Build history of the part. All positions in model axes, mm. Round coordinates to 2 decimals unless told otherwise and drop trailing zeros. Loops run counter-clockwise (first coordinate to the right, second up) from the corner with the lowest first, then second, coordinate; pieces in that order, holes last. Notation, with made-up numbers: (72, 20) - (110, 20) arc R28 cw to (110, 43) - close; hole circle Ø2 at (70.5, -6.5). An arc over 180 degrees is marked (long way). Use a Markdown table: item, result.
from build123d import *

# Parameters (mm, degrees)
F0_W     = 254
F0_H     = 254
F1_DEPTH = 162.56
F2_R     = 60.882574
F3_DEPTH = 289.56
F4_SIZE  = 5.08
F5_R     = 12.7
F6_R     = 12.7


with BuildPart() as f1:
    # F0 (on Top) → F1 (new body)
    with BuildSketch(Plane.XY):
        Rectangle(F0_W, F0_H)
    extrude(amount=F1_DEPTH)

    # F2 (on face) → F3 (cut)
    with BuildSketch(Plane.XY.offset(162.56)):
        Circle(F2_R)
    extrude(amount=-F3_DEPTH, mode=Mode.SUBTRACT)

    # F4
    f4_edges = [f1.edges().sort_by_distance(p)[0] for p in [
        (127, 0, 162.56),
        (0, -127, 162.56),
        (-127, 0, 162.56),
        (0, 127, 162.56),
        (-60.882574, 0, 162.56),
    ]]
    chamfer(f4_edges, length=F4_SIZE)

    # F5
    f5_edges = [f1.edges().sort_by_distance(p)[0] for p in [
        (-127, 0, 0),
        (0, 127, 0),
        (127, 0, 0),
        (0, -127, 0),
    ]]
    fillet(f5_edges, radius=F5_R)

    # F6
    f6_edges = [f1.edges().sort_by_distance(p)[0] for p in [
        (-60.882574, 0, 0),
    ]]
    fillet(f6_edges, radius=F6_R)


solid = f1.part
Q1. Cut at A-A, the plane x = 0. List the corners of the cut face in (y, z).
Results found:
| item | result |
|---|---|
| outline | (-127, 12.7) arc R12.7 ccw to (-114.3, 0) - (-73.58, 0) arc R12.7 ccw to (-60.88, 12.7) - (-60.88, 157.48) - (-65.96, 162.56) - (-121.92, 162.56) - (-127, 157.48) - close; (60.88, 12.7) arc R12.7 ccw to (73.58, 0) - (114.3, 0) arc R12.7 ccw to (127, 12.7) - (127, 157.48) - (121.92, 162.56) - (65.96, 162.56) - (60.88, 157.48) - close |
Q2. Pull direction X, two halves, no side cores. Call faces 1 (the face through (52, 56, 162.56)), 2 (the face through (-13.198, -59.435, 86.103)), 3 (the face through (-13.25, -59.68, 157.73)), 4 (the face through (-127, -2, 84)): pulls with the +X half, pulls with the -X half, needs draft (parallel to the pull), parting line crosses it, or undercut.
Results found:
| item | result |
|---|---|
| face 1 | needs draft |
| face 2 | undercut |
| face 3 | undercut |
| face 4 | pulls with the -X half |
Q3. Drop a flat-ended pin along its axis: pin 1 (2 mm diameter, centred on x = -60.5, y = -14, fed in from -Z). Give the stop position or say it passes through.
Results found:
| item | result |
|---|---|
| pin 1 | stops at z = 5.53 |
Q4. Cut at C-C, the plane z = 128.5. List the corners of the cut face in (x, y), plus the area to 3 significant figures.
Results found:
| item | result |
|---|---|
| outline | (-127, -127) - (127, -127) - (127, 127) - (-127, 127) - close; hole circle Ø121.77 at (0, 0) |
| area | 52,900 mm2 |
Q5. Probe line 1 (Y direction, x = 0, z = 57); line 2 (Y direction, x = 36, z = 85); line 3 (X direction, y = -22, z = 23.5). List the from-to ranges inside material, lowest first.
Results found:
| item | result |
|---|---|
| line 1 | y = -127 to -60.88, 60.88 to 127 |
| line 2 | y = -127 to -49.1, 49.1 to 127 |
| line 3 | x = -127 to -56.77, 56.77 to 127 |
